from build123d import *

# Parameters (mm, degrees)
SKETCH1_W           = 20
SKETCH1_H           = 10
BOSS_EXTRUDE1_DEPTH = 6
SKETCH2_W           = 0.5
SKETCH2_H           = 3
BOSS_EXTRUDE2_DEPTH = 4
SKETCH3_R           = 1.25
CUT_EXTRUDE1_DEPTH  = 15.730919863


with BuildPart() as part:
    # Sketch1 → Boss-Extrude1 (new body)
    with BuildSketch(Plane.XY):
        Rectangle(SKETCH1_W, SKETCH1_H)
    extrude(amount=BOSS_EXTRUDE1_DEPTH)

    # Sketch2 → Boss-Extrude2 (add)
    with BuildSketch(Plane(origin=(0, 5, 0), x_dir=(1, 0, 0), z_dir=(0, 1, 0))):
        with Locations((-8.212529155, -3)):
            Rectangle(SKETCH2_W, SKETCH2_H)
        with Locations((0.087470845, -3)):
            Rectangle(SKETCH2_W, SKETCH2_H)
        with Locations((8.387470845, -3)):
            Rectangle(SKETCH2_W, SKETCH2_H)
    extrude(amount=BOSS_EXTRUDE2_DEPTH)

    # Sketch3 → Cut-Extrude1 (cut, through all)
    with BuildSketch(Plane.XY.offset(6)):
        with Locations((-4.75, 2)):
            Circle(SKETCH3_R)
        with Locations((4.75, 2)):
            Circle(SKETCH3_R)
    extrude(amount=-CUT_EXTRUDE1_DEPTH, mode=Mode.SUBTRACT)


solid = part.part
Check sheet for the modelled part. Datum: model origin and axes. Units: mm. A direction names the side the tool comes from. Give positions to 0.01 mm unless a question says otherwise; leave off trailing zeros. Loops run counter-clockwise (first coordinate to the right, second up) from the corner with the lowest first, then second, coordinate; pieces in that order, holes last. Notation, with made-up numbers: M 72.5,4.5 L 130.5,4.5 A16 cw 130.5,35.5 Z; hole C 30,50.5 d6. An arc over 180 degrees is marked long. Use a Markdown table: item, result. Add a question column.
Q1. Tool access check on faces 1 (the flat face through (-8.463, 7, 3)), 2 (the flat face through (8.637, 7, 3)), 3 (the flat face through (0, 0, 6)), 4 (the flat face through (-7.963, 7, 3)). Record the directions out of +Z, -Z, +X, -X, +Y, -Y that give a thin tool (end or side, any length) a straight path to the whole face; none if there is none.
Q2. Go/stop test with flat-tipped pins: pin 1 (2 mm diameter, centred on x = -4.75, y = 2, fed in from +Z); pin 2 (1.5 mm diameter, centred on y = 6, z = 3.5, fed in from +X); pin 3 (1.5 mm diameter, centred on y = 6.5, z = 3.5, fed in from -X). Record where each tip stops, or that it passes through.
Q3. Sectioned sample at D-D, the plane x = 3.75. Record the cut outline in (y, z).
Q4. Mould release check, pull along X, two halves, no side actions. Record for faces 5 (the cylindrical face through (4.59, 3.24, 3.04)), 6 (the flat face through (0, 5, 1)), 7 (the flat face through (-10, 0, 3)), 8 (the flat face through (10, 0, 3)): pulls with the +X half, pulls with the -X half, needs draft (parallel to the pull), parting line crosses it, or undercut.
Q5. Sectioned sample at C-C, the plane z = 1.05. Record the cut outline in (x, y), then the cut area to 3 significant figures.
Q6. Sectioned sample at A-A, the plane x = -4.75. Record the cut outline in (y, z).
Q7. Scan lines: line 1 along Y through (x, z) = (-4.75, 2.05); line 2 along X through (y, z) = (2.5, 2.7); line 3 along Y through (x, z) = (-7.5, 5.35). Record each from-to range of solid material in increasing order. Write a range as [from, to].
Q8. Sectioned sample at B-B, the plane y = 2. Record the cut outline in (x, z), then the cut area to 3 significant figures.
Verdict:
| question | item | result |
|---|---|---|
| 1 | face 1 | +Z, -Z, -X, +Y |
| 1 | face 2 | +Z, -Z, +X, +Y |
| 1 | face 3 | +Z, +X, -X, +Y, -Y |
| 1 | face 4 | +Z, -Z, +Y |
| 2 | pin 1 | through |
| 2 | pin 2 | x = 8.64 |
| 2 | pin 3 | x = -8.46 |
| 3 | outline | M -5,0 L 1.25,0 L 1.25,6 L -5,6 Z; M 2.75,0 L 5,0 L 5,6 L 2.75,6 Z |
| 4 | face 5 | undercut |
| 4 | face 6 | undercut |
| 4 | face 7 | pulls with the -X half |
| 4 | face 8 | pulls with the +X half |
| 5 | outline | M -10,-5 L 10,-5 L 10,5 L -10,5 Z; hole C -4.75,2 d2.5; hole C 4.75,2 d2.5 |
| 5 | area | 190 mm^2 |
| 6 | outline | M -5,0 L 0.75,0 L 0.75,6 L -5,6 Z; M 3.25,0 L 5,0 L 5,6 L 3.25,6 Z |
| 7 | line 1 | [-5, 0.75], [3.25, 5] |
| 7 | line 2 | [-10, -5.9], [-3.6, 3.6], [5.9, 10] |
| 7 | line 3 | [-5, 5] |
| 8 | outline | M -10,0 L -6,0 L -6,6 L -10,6 Z; M -3.5,0 L 3.5,0 L 3.5,6 L -3.5,6 Z; M 6,0 L 10,0 L 10,6 L 6,6 Z |
| 8 | area | 90.0 mm^2 |
